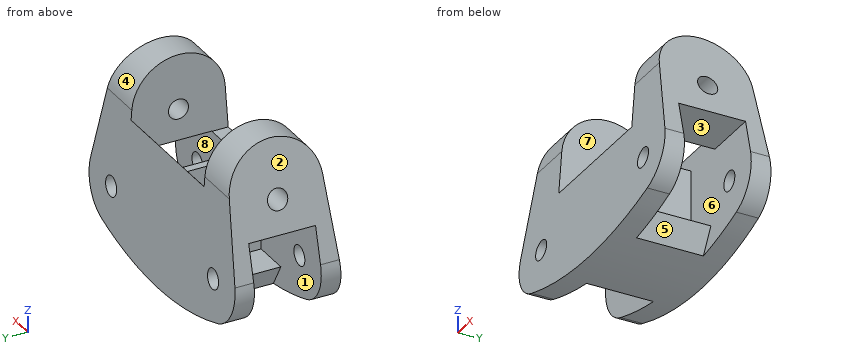
from build123d import *

# Parameters (mm, degrees)
SKETCH1_R          = 1.5
EXTRUDE1_DEPTH     = 8.5
SKETCH2_R          = 1.5
CUT_EXTRUDE1_DEPTH = 25
CUT_EXTRUDE2_DEPTH = 10
CUT_EXTRUDE3_DEPTH = 5


with BuildPart() as part:
    # Sketch1 → Extrude1 (new, symmetric)
    with BuildSketch(Plane(origin=(0, 0, 0), x_dir=(1, 0, 0), z_dir=(0, 1, 0))):
        with BuildLine():
            Line((-15, 0), (15, 0))
            Line((15, 0), (19.755405538, 18.21438149))
            ThreePointArc((19.755405538, 18.21438149), (19.225810264, 22.587646069), (15.852272727, 25.420517177))
            ThreePointArc((15.852272727, 25.420517177), (0, 28), (-15.852272727, 25.420517177))
            ThreePointArc((-15.852272727, 25.420517177), (-19.225810264, 22.587646069), (-19.755405538, 18.21438149))
            Line((-19.755405538, 18.21438149), (-15, 0))
        make_face()
        with Locations(Location((-13.95, 19.730055116, 0), (0, 0, 270))):
            Circle(SKETCH1_R, mode=Mode.SUBTRACT)
        with Locations(Location((13.95, 19.730055116, 0), (0, 0, 270))):
            Circle(SKETCH1_R, mode=Mode.SUBTRACT)
    extrude(amount=EXTRUDE1_DEPTH, both=True)

    # Sketch2 → Cut-Extrude1 (cut, symmetric)
    with BuildSketch(Plane(origin=(0, 0, 0), x_dir=(0, 0, -1), z_dir=(1, 0, 0))):
        with Locations((8.255055116, 0)):
            Circle(SKETCH2_R)
        with BuildLine():
            Line((6.507034671, 6.982620223), (29, 8.570598903))
            Line((29, 8.570598903), (29, 9.570598903))
            Line((29, 9.570598903), (-1, 9.570598903))
            Line((-1, 9.570598903), (-1, -9.570598903))
            Line((-1, -9.570598903), (29, -9.570598903))
            Line((29, -9.570598903), (29, -8.570598903))
            Line((29, -8.570598903), (6.507034671, -6.982620223))
            ThreePointArc((6.507034671, -6.982620223), (0, 0), (6.507034671, 6.982620223))
        make_face()
    extrude(amount=CUT_EXTRUDE1_DEPTH, both=True, mode=Mode.SUBTRACT)

    # Sketch4 → Cut-Extrude2 (cut, symmetric)
    with BuildSketch(Plane(origin=(0, 0, 0), x_dir=(0, 0, -1), z_dir=(1, 0, 0))):
        Polygon((-2, -8.5), (13, -8.5), (13, 5), (10.488407646, 5), (5.125516479, 9.5), (-2, 9.5), align=None)
    extrude(amount=CUT_EXTRUDE2_DEPTH, both=True, mode=Mode.SUBTRACT)

    # Sketch7 → Cut-Extrude3 (cut, symmetric)
    with BuildSketch(Plane(origin=(0, 0, 0), x_dir=(1, 0, 0), z_dir=(0, 1, 0))):
        Polygon((-10, 6.507034671), (-10, 12.951116752), (-21.755405538, 12.951116752), (-21.755405538, 29), (-6, 29), (-8.886751346, 24), (-3.5, 24), (-3.5, 8), (-2.25, 8), (-2.25, 24), (2.25, 24), (2.25, 8), (3.5, 8), (3.5, 24), (8.886751346, 24), (6, 29), (21.755405538, 29), (21.755405538, 12.951116752), (10, 12.951116752), (10, 6.507034671), align=None)
    extrude(amount=CUT_EXTRUDE3_DEPTH, both=True, mode=Mode.SUBTRACT)


solid = part.part
Part model, mm, in its own coordinate system. Face numbers are marked on the shaded views. A direction names the side the tool comes from. Give positions to 0.01 mm unless a question says otherwise; leave off trailing zeros. Loops run counter-clockwise (first coordinate to the right, second up) from the corner with the lowest first, then second, coordinate; pieces in that order, holes last. Notation, with made-up numbers: M -39,73.5 L -15,73.5 A23 cw -15,81.5 Z; hole C 10.25,15 d5. An arc over 180 degrees is marked long. Put each result on its own line as item: value. Start each with the question number.
1) Saw through at D-D (z = -2.25). List the corners of the cut face in (x, y), then the cut area to 3 significant figures.
2) Saw through at A-A (x = 13.95). List the corners of the cut face in (y, z), then the cut area to 3 significant figures.
3) Pull direction Y, two halves, no side cores. Call the marked faces 1, 2, 3 and 4: +Y half, -Y half, draft (parallel to the pull), parting line (faces both ways), or undercut.
4) 3-axis set-ups, long thin cutter, end or side, ignore diameter. For the marked faces 5, 6, 7 and 8: which of +Z, -Z, +X, -X, +Y, -Y reach the whole face in a straight line?
5) Flat gauge pins, fed straight in: pin 1 (5 mm diameter, centred on y = -7, z = -10, fed in from +X); pin 2 (8 mm diameter, centred on y = -3.5, z = -15.5, fed in from +X); pin 3 (2.5 mm diameter, centred on x = -7, y = -1, fed in from +Z). Where does each tip first touch, or does it go through?
6) Saw through at B-B (y = 4.25). List the corners of the cut face in (x, z), then the cut area to 3 significant figures.
7) Probe probe 1 along X at (y, z) = (3.25, -13.75); probe 2 along X at (y, z) = (5.5, -20.75); probe 3 along Z at (x, y) = (-12, 0). List the from-to ranges inside material, lowest first.
8) Saw through at C-C (y = 0). List the corners of the cut face in (x, z).
Numbers:
1. outline: M -15.59,-5.14 L -10,-5.14 L -10,5.14 L -15.59,5.14 Z; M 10,-5.14 L 15.59,-5.14 L 15.59,5.14 L 10,5.14 Z
1. area: 115 mm^2
2. outline: M -8.36,-26.01 L -5,-26.01 L -5,-21.23 L -8.02,-21.23 Z; M -7.81,-18.23 L -5,-18.23 L -5,-12.95 L 5,-12.95 L 5,-18.23 L 7.81,-18.23 L 6.98,-6.51 A7 ccw -6.98,-6.51 Z; M 5,-26.01 L 8.36,-26.01 L 8.02,-21.23 L 5,-21.23 Z; hole C 0,-8.26 d3
2. area: 214 mm^2
3. face 1: undercut
3. face 2: draft
3. face 3: undercut
3. face 4: parting line
4. face 5: -Z, +X
4. face 6: none
4. face 7: +Z, -Y
4. face 8: +X
5. pin 1: x = 18.26
5. pin 2: x = 19.93
5. pin 3: z = -24
6. outline: M -18.38,-12.95 L -10,-12.95 L -10,-1.44 L -15.38,-1.44 Z; M -8.89,-24 L -6.85,-27.53 A50 ccw 6.85,-27.53 L 8.89,-24 L 3.5,-24 L 3.5,-13 L 2.25,-13 L 2.25,-24 L -2.25,-24 L -2.25,-13 L -3.5,-13 L -3.5,-24 Z; M 10,-12.95 L 18.38,-12.95 L 15.38,-1.44 L 10,-1.44 Z
6. area: 246 mm^2
7. probe 1: -3.5 to -2.25, 2.25 to 3.5
7. probe 2: -19.86 to -15.05, -12.85 to 12.85, 15.05 to 19.86
7. probe 3: -12.95 to -9.76, -6.76 to 0
8. outline: M -18.38,-12.95 L -10,-12.95 L -10,-9.76 L -17.55,-9.76 Z; M -16.76,-6.76 L -10,-6.76 L -10,0 L -15,0 Z; M -8.89,-24 L -6.85,-27.53 A50 ccw 6.85,-27.53 L 8.89,-24 L 3.5,-24 L 3.5,-13 L 2.25,-13 L 2.25,-24 L -2.25,-24 L -2.25,-13 L -3.5,-13 L -3.5,-24 Z; M 10,-12.95 L 18.38,-12.95 L 17.55,-9.76 L 10,-9.76 Z; M 10,-6.76 L 16.76,-6.76 L 15,0 L 10,0 Z
